from build123d import *

# Parameters (mm, degrees)
SKETCH1_W               = 34
SKETCH1_H               = 14
BOSS_EXTRUDE1_DEPTH     = 10
SKETCH2_R               = 8.1
CUT_EXTRUDE1_DEPTH      = 4
CUT_EXTRUDE2_DEPTH      = 39.105117767
CUT_EXTRUDE2_DEPTH_BACK = 39.105117767
SKETCH4_R               = 6.1
CUT_EXTRUDE3_DEPTH      = 39.105117767
CUT_EXTRUDE3_DEPTH_BACK = 39.105117767
SKETCH5_R               = 1.8
CUT_EXTRUDE4_DEPTH      = 2.4
CHAMFER1_SIZE           = 3


with BuildPart() as part:
    # Sketch1 → Boss-Extrude1 (new body)
    with BuildSketch(Plane(origin=(0, 0, 0), x_dir=(1, 0, 0), z_dir=(0, 1, 0))):
        with Locations((17, 7)):
            Rectangle(SKETCH1_W, SKETCH1_H)
    extrude(amount=BOSS_EXTRUDE1_DEPTH)

    # Sketch2 → Cut-Extrude1 (cut)
    with BuildSketch(Plane(origin=(0, 10, 0), x_dir=(1, 0, 0), z_dir=(0, 1, 0))):
        with Locations((17, 14)):
            Circle(SKETCH2_R)
    extrude(amount=-CUT_EXTRUDE1_DEPTH, mode=Mode.SUBTRACT)

    # Sketch4 → Cut-Extrude2 (cut, two sides: drawn at the far end of the back side and taken through both)
    with BuildSketch(Plane(origin=(0, 10, 0), x_dir=(1, 0, 0), z_dir=(0, 1, 0)).offset(-CUT_EXTRUDE2_DEPTH_BACK)):
        with Locations((17, 14)):
            Circle(SKETCH4_R)
    extrude(amount=CUT_EXTRUDE2_DEPTH + CUT_EXTRUDE2_DEPTH_BACK, mode=Mode.SUBTRACT)

    # Sketch5 → Cut-Extrude3 (cut, two sides: drawn at the far end of the back side and taken through both)
    with BuildSketch(Plane(origin=(0, 0, -14), x_dir=(-1, 0, 0), z_dir=(0, 0, -1)).offset(-CUT_EXTRUDE3_DEPTH_BACK)):
        with Locations((-29, 5)):
            Circle(SKETCH5_R)
        with Locations((-5, 5)):
            Circle(SKETCH5_R)
    extrude(amount=CUT_EXTRUDE3_DEPTH + CUT_EXTRUDE3_DEPTH_BACK, mode=Mode.SUBTRACT)

    # Sketch6 → Cut-Extrude4 (cut)
    with BuildSketch(Plane.XY):
        Polygon((8.290896534, 5), (6.645448267, 7.85), (3.354551733, 7.85), (1.709103466, 5), (3.354551733, 2.15), (6.645448267, 2.15), align=None)
        Polygon((25.709103466, 5), (27.354551733, 2.15), (30.645448267, 2.15), (32.290896534, 5), (30.645448267, 7.85), (27.354551733, 7.85), align=None)
    extrude(amount=-CUT_EXTRUDE4_DEPTH, mode=Mode.SUBTRACT)

    # Chamfer1
    chamfer1_edges = [part.edges().sort_by_distance(p)[0] for p in [
        (34, 0, -7),
        (0, 0, -7),
    ]]
    chamfer(chamfer1_edges, length=CHAMFER1_SIZE)


solid = part.part
Verification items for the finished model (mm, model axes). A direction names the side the tool comes from. Give positions to 0.01 mm unless a question says otherwise; leave off trailing zeros. Loops run counter-clockwise (first coordinate to the right, second up) from the corner with the lowest first, then second, coordinate; pieces in that order, holes last. Notation, with made-up numbers: (-28.75, -11) - (24.25, -11) arc R14 ccw to (24.25, 8) - close; hole circle Ø1 at (56, 89.25). An arc over 180 degrees is marked (long way). Write each question's results on one line, items separated by ' | '.
1) Sectioned sample at A-A on x = 5. Record the boundary of the cut face in (y, z).
Solution:
outline: (0, -14) - (3.2, -14) - (3.2, -2.4) - (2.15, -2.4) - (2.15, 0) - (0, 0) - close; (6.8, -14) - (10, -14) - (10, 0) - (7.85, 0) - (7.85, -2.4) - (6.8, -2.4) - close
2) Sectioned sample at C-C on z = -7. Record the boundary of the cut face in (x, y).
Solution:
outline: (0, 3) - (3, 0) - (31, 0) - (34, 3) - (34, 10) - (21.08, 10) - (21.08, 6) - (12.92, 6) - (12.92, 10) - (0, 10) - close; hole circle Ø3.6 at (5, 5); hole circle Ø3.6 at (29, 5)
3) Mould release check, pull along Y, two halves, no side actions. Record for faces 1 (the cylindrical face through (16.82, 8.03, -5.9)), 2 (the flat face through (26.52, 3.595, -1.183)), 3 (the flat face through (33, 2, -7)): pulls with the +Y half, pulls with the -Y half, needs draft (parallel to the pull), parting line crosses it, or undercut.
Solution:
face 1: needs draft | face 2: undercut | face 3: pulls with the -Y half
4) Sectioned sample at D-D on y = 1. Record the boundary of the cut face in (x, z), plus the area to 3 significant figures.
Solution:
outline: (2, -14) - (10.9, -14) arc R6.1 cw to (23.1, -14) - (32, -14) - (32, 0) - (2, 0) - close | area: 362 mm2
5) Depth check by flat-ended pin: P1, Ø3, axis at x = 30, y = 4.5, coming from the +Z side; P2, Ø2.5, axis at x = 19, z = -8.5, coming from the +Y side; P3, Ø5, axis at x = 15.5, z = -9, coming from the -Y side; P4, Ø1.5, axis at x = 17.5, y = 3, coming from the -Z side. Enter the tip coordinate at first touch or a pass-through.
Solution:
P1: z = -2.4 | P2: y = 6 | P3: y = 0 | P4: z = -8.03
6) Tool access check on faces 4 (the cylindrical face through (27.337, 4.311, -8.119)), 5 (the flat face through (5, 7.85, -1)), 6 (the flat face through (17, 6, -7.6)). Record the directions out of +Z, -Z, +X, -X, +Y, -Y that give a thin tool (end or side, any length) a straight path to the whole face; none if there is none.
Solution:
face 4: +Z, -Z | face 5: +Z | face 6: -Z, +Y
7) Sectioned sample at B-B on z = -9.75. Record the boundary of the cut face in (x, y), plus the area to 3 significant figures.
Solution:
outline: (0, 3) - (3, 0) - (12.62, 0) - (12.62, 6) - (10.1, 6) - (10.1, 10) - (0, 10) - close; (21.38, 0) - (31, 0) - (34, 3) - (34, 10) - (23.9, 10) - (23.9, 6) - (21.38, 6) - close; hole circle Ø3.6 at (5, 5); hole circle Ø3.6 at (29, 5) | area: 203 mm2
8) Material ranges on L1, parallel to X at y = 5, z = -6; L2, parallel to Y at x = 5, z = -10.5; L3, parallel to X at y = 6, z = -2.5, recorded low to high. Write a range as from..to.
Solution:
L1: 0..3.2, 6.8..27.2, 30.8..34 | L2: 0..3.2, 6.8..10 | L3: 0..3.5, 6.5..27.5, 30.5..34
